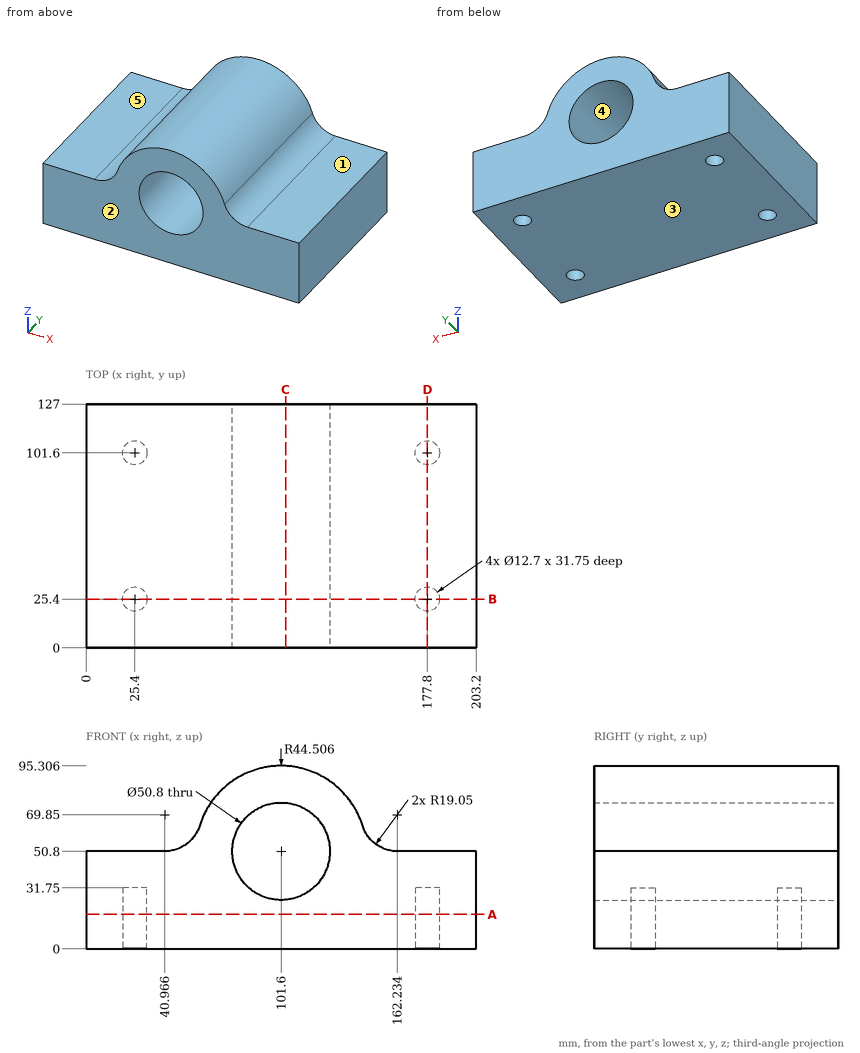
Answer from the drawing. Dimensions are ordinates in mm from the lowest x, y and z of the part. A direction names the side the tool comes from. Coordinates: 2 decimals unless noted, no trailing zeros. Write each loop counter-clockwise with the first axis right and the second up, starting at its lowest first coordinate (ties: lowest second). Pieces come first, ordered by that corner, then holes. Notation, with made-up numbers: (84.25, 77.5) - (110.25, 77.5) arc R37 cw to (110.25, 114.5) - close; hole circle Ø10 at (59.25, 1). An arc over 180 degrees is marked (long way). Return JSON: item names as keys, results as strings. Group by question number.
Q1. Flat-ended cylindrical pins translate along their axes: pin 1 Ø4 at (x, y) = (24.5, 28) entering from -Z; pin 2 Ø12.5 at (x, y) = (180.5, 87) entering from +Z. Find the tip coordinate at first contact, or state that the pin passes through.
Q2. Which of the six approach directions +Z, -Z, +X, -X, +Y, -Y give full straight-line access (tool end or side, diameter ignored) to the marked faces 1 and 2?
Q3. The part is cut by section D-D on x = 177.8. Write down the section's boundary in (y, z), and give its area (4 significant figures).
Q4. The part is cut by section A-A on z = 18. Write down the section's boundary in (x, y), and give its area (3 significant figures).
Q5. The part is cut by section B-B on y = 25.4. Write down the section's boundary in (x, z), and give its area (3 significant figures).
Q6. Find the intervals of material crossed by line 1 along X through (y, z) = (25, 17); line 2 along Y through (x, z) = (25.4, 15.5); line 3 along X through (y, z) = (78, 50), in increasing order. Write a range as [from, to].
Q7. The part is cut by section C-C on x = 104. Write down the section's boundary in (y, z), and give its area (3 significant figures).
Q8. For a pull along Z with two mould halves and no side action, classify the marked faces 3, 4 and 5 as +Z half, -Z half, draft (parallel to the pull), parting line (faces both ways), or undercut.
Evaluation:
{
 "1": {"pin 1": "stops at z = 31.75", "pin 2": "stops at z = 50.8"},
 "2": {"face 1": "+Z, +X, +Y, -Y", "face 2": "+Z, -Z, +X, -X, -Y"},
 "3": {"outline": "(0, 0) - (19.05, 0) - (19.05, 31.75) - (31.75, 31.75) - (31.75, 0) - (95.25, 0) - (95.25, 31.75) - (107.95, 31.75) - (107.95, 0) - (127, 0) - (127, 50.8) - (0, 50.8) - close", "area": "5,645 mm2"},
 "4": {"outline": "(0, 0) - (203.2, 0) - (203.2, 127) - (0, 127) - close; hole circle Ø12.7 at (25.4, 25.4); hole circle Ø12.7 at (25.4, 101.6); hole circle Ø12.7 at (177.8, 25.4); hole circle Ø12.7 at (177.8, 101.6)", "area": "25,300 mm2"},
 "5": {"outline": "(0, 0) - (19.05, 0) - (19.05, 31.75) - (31.75, 31.75) - (31.75, 0) - (171.45, 0) - (171.45, 31.75) - (184.15, 31.75) - (184.15, 0) - (203.2, 0) - (203.2, 50.8) - (162.23, 50.8) arc R19.05 cw to (144.06, 64.14) arc R44.51 ccw to (59.14, 64.14) arc R19.05 cw to (40.97, 50.8) - (0, 50.8) - close; hole circle Ø50.8 at (101.6, 50.8)", "area": "10,700 mm2"},
 "6": {"line 1": "x = [0, 19.06], [31.74, 171.46], [184.14, 203.2]", "line 2": "y = [0, 19.05], [31.75, 95.25], [107.95, 127]", "line 3": "x = [0, 76.21], [126.99, 203.2]"},
 "7": {"outline": "(0, 0) - (127, 0) - (127, 25.51) - (0, 25.51) - close; (0, 76.09) - (127, 76.09) - (127, 95.24) - (0, 95.24) - close", "area": "5,670 mm2"},
 "8": {"face 3": "-Z half", "face 4": "undercut", "face 5": "+Z half"}
}
